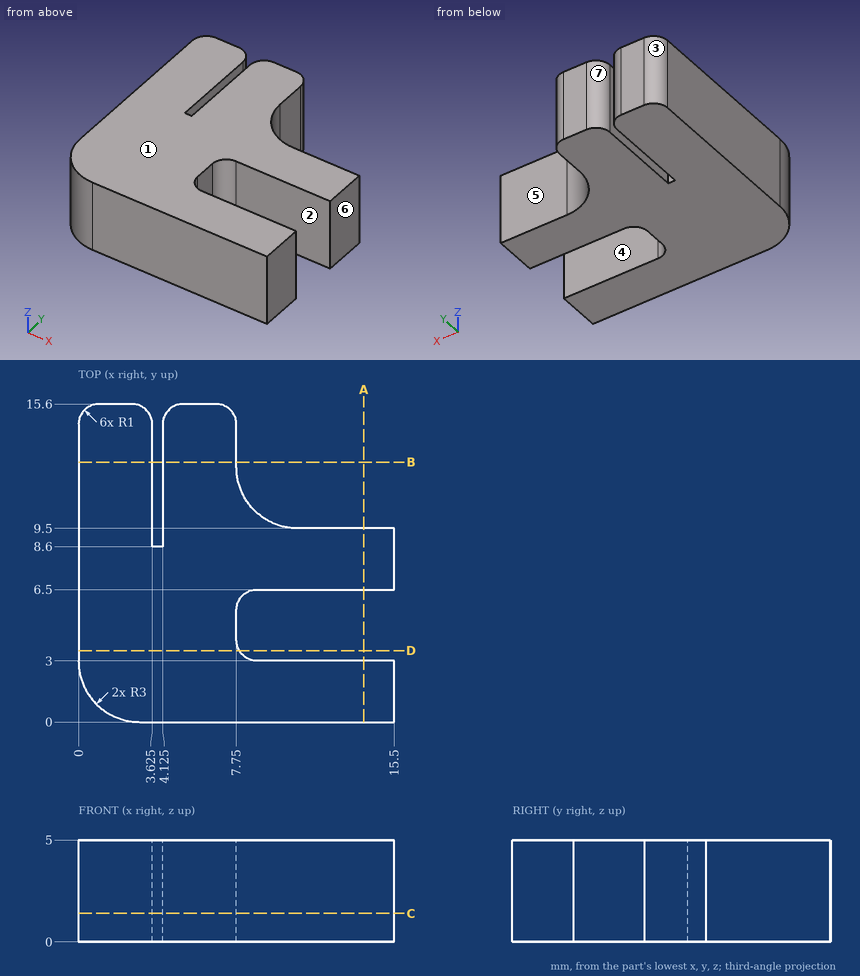
Could you check a few things on this drawing? It's one solid part, dimensions in mm from its lowest x, y, z. A direction names the side the tool comes from. Coordinates: 2 decimals unless noted, no trailing zeros. Order: outer loops, then holes, each group sorted by start corner. A loop starts at its lowest first (then second) coordinate and runs counter-clockwise, first axis right, second up.
1. Thinking about a two-plate mould opening in Y: for the marked faces 1, 2 and 3, which applies, +Y half, -Y half, draft (parallel to the pull), parting line (faces both ways), or undercut?
2. For the marked faces 4, 5, 6 and 7, which set-ups out of +Z, -Z, +X, -X, +Y, -Y let a thin tool reach every point of the face, with its end or its side?
3. I need wall thicknesses on line 1 (Y direction, x = 13.5, z = 3.5); line 2 (X direction, y = 14.25, z = 1.65) (3 decimals); line 3 (Y direction, x = 8, z = 3.6). Which ranges of each line are inside material? Lowest first, please.
4. I'm going to push flat-ended pins straight in: pin 1 (1.5 mm diameter, centred on x = 12, z = 2, fed in from +Y); pin 2 (1.7 mm diameter, centred on y = 13.5, z = 3.5, fed in from +X); pin 3 (2.5 mm diameter, centred on y = 11.5, z = 2, fed in from +X). Where does each tip first touch, or does it pass through?
5. If we section it at D-D (y = 3.5): Please give me the cut outline in (x, z).
6. If we section it at C-C (z = 1.4): Please give me the cut outline in (x, y) (3 decimals).
7. If we section it at B-B (y = 12.75): Please give me the cut outline in (x, z) (3 decimals), then the cut area to 4 significant figures.
8. If we section it at A-A (x = 14): Please give me the cut outline in (y, z), then the cut area to 3 significant figures.
Entries:
1. face 1: draft
1. face 2: undercut
1. face 3: +Y half
2. face 4: +Z, -Z, +X
2. face 5: +Z, -Z, +X, +Y
2. face 6: +Z, -Z, +X, +Y, -Y
2. face 7: +Z, -Z, +Y
3. line 1: y = 0 to 3, 6.5 to 9.5
3. line 2: x = 0 to 3.625, 4.125 to 7.75
3. line 3: y = 0 to 3.34, 6.16 to 11.3
4. pin 1: stops at y = 9.5
4. pin 2: stops at x = 7.75
4. pin 3: stops at x = 8.77
5. outline: (0, 0) - (7.88, 0) - (7.88, 5) - (0, 5) - close
6. outline: (0, 3) arc R3 ccw to (3, 0) - (15.5, 0) - (15.5, 3) - (8.75, 3) arc R1 cw to (7.75, 4) - (7.75, 5.5) arc R1 cw to (8.75, 6.5) - (15.5, 6.5) - (15.5, 9.5) - (10.75, 9.5) arc R3 cw to (7.75, 12.5) - (7.75, 14.6) arc R1 ccw to (6.75, 15.6) - (5.125, 15.6) arc R1 ccw to (4.125, 14.6) - (4.125, 8.6) - (3.625, 8.6) - (3.625, 14.6) arc R1 ccw to (2.625, 15.6) - (1, 15.6) arc R1 ccw to (0, 14.6) - close
7. outline: (0, 0) - (3.625, 0) - (3.625, 5) - (0, 5) - close; (4.125, 0) - (7.75, 0) - (7.75, 5) - (4.125, 5) - close
7. area: 36.25 mm2
8. outline: (0, 0) - (3, 0) - (3, 5) - (0, 5) - close; (6.5, 0) - (9.5, 0) - (9.5, 5) - (6.5, 5) - close
8. area: 30.0 mm2
